```python
from build123d import *

# Parameters (mm, degrees)
BOSS_EXTRUDE1_DEPTH = 0.254
SKETCH2_R           = 4.699
CUT_EXTRUDE1_DEPTH  = 1.254
SKETCH3_W           = 2.54
SKETCH3_H           = 0.635
CUT_EXTRUDE2_DEPTH  = 1.254
CUT_EXTRUDE4_DEPTH  = 1.254
CUT_EXTRUDE5_DEPTH  = 1.254


with BuildPart() as part:
    # Sketch1 → Boss-Extrude1 (new body)
    with BuildSketch(Plane.XY):
        with BuildLine():
            Line((67.21146711, 76.191723231), (8.696654013, 17.676910134))
            Line((8.696654013, 17.676910134), (7.228954972, 14.133571205))
            ThreePointArc((7.228954972, 14.133571205), (14.666587579, 6.075099489), (15.105587123, -4.88230096))
            Line((15.105587123, -4.88230096), (18.648926052, -6.35))
            Line((18.648926052, -6.35), (101.401368334, -6.35))
            ThreePointArc((101.401368334, -6.35), (93.866160503, 38.880636728), (67.21146711, 76.191723231))
        make_face()
        with BuildLine():
            Line((88.672924278, 6.35), (27.86051193, 6.35))
            ThreePointArc((27.86051193, 6.35), (26.399857642, 10.93517908), (24.190484974, 15.210228852))
            Line((24.190484974, 15.210228852), (67.191354125, 58.211098004))
            ThreePointArc((67.191354125, 58.211098004), (82.13289044, 34.020557137), (88.672924278, 6.35))
        make_face(mode=Mode.SUBTRACT)
    extrude(amount=BOSS_EXTRUDE1_DEPTH)

    # Sketch2 → Cut-Extrude1 (cut, through all)
    with BuildSketch(Plane.XY.offset(0.254)):
        with Locations((22.225, 0)):
            Circle(SKETCH2_R)
        with Locations((36.195, 0)):
            Circle(SKETCH2_R)
        with Locations((61.722, 0)):
            Circle(SKETCH2_R)
        with Locations((75.692, 0)):
            Circle(SKETCH2_R)
        with Locations((95.25, 0)):
            Circle(SKETCH2_R)
        with Locations((15.715448212, 15.715448212)):
            Circle(SKETCH2_R)
        with Locations((25.593729945, 25.593729945)):
            Circle(SKETCH2_R)
        with Locations((43.644044748, 43.644044748)):
            Circle(SKETCH2_R)
        with Locations((53.522326482, 53.522326482)):
            Circle(SKETCH2_R)
        with Locations((92.004434954, 24.652514046)):
            Circle(SKETCH2_R)
        with Locations((82.48891971, 47.625)):
            Circle(SKETCH2_R)
        with Locations((67.351920908, 67.351920908)):
            Circle(SKETCH2_R)
    extrude(amount=-CUT_EXTRUDE1_DEPTH, mode=Mode.SUBTRACT)

    # Sketch3 → Cut-Extrude2 (cut, through all)
    with BuildSketch(Plane.XY.offset(0.254)):
        Polygon((15.266435406, 24.246691527), (17.06248663, 26.042742751), (17.511499436, 25.593729945), (15.715448212, 23.797678721), align=None)
        Polygon((44.991083167, 53.971339288), (43.195031942, 52.175288063), (43.644044748, 51.726275257), (45.440095973, 53.522326482), align=None)
        with Locations((29.21, -6.0325)):
            Rectangle(SKETCH3_W, SKETCH3_H)
        with Locations((68.707, -6.0325)):
            Rectangle(SKETCH3_W, SKETCH3_H)
        Polygon((29.230733674, 38.210989795), (31.026784898, 40.007041019), (31.475797704, 39.558028213), (29.67974648, 37.761976989), align=None)
        Polygon((56.845021246, 65.825277367), (55.048970022, 64.029226143), (55.497982828, 63.580213337), (57.294034052, 65.376264561), align=None)
        with Locations((48.9585, -6.0325)):
            Rectangle(SKETCH3_W, SKETCH3_H)
        with Locations((85.471, -6.0325)):
            Rectangle(SKETCH3_W, SKETCH3_H)
        Polygon((99.935462164, 14.437711971), (100.266998693, 11.919442024), (101.526133667, 12.085210288), (101.194597138, 14.603480236), align=None)
        Polygon((93.765504959, 37.464305742), (94.938831965, 37.950313702), (93.966816047, 40.296967714), (92.793489041, 39.810959755), align=None)
        Polygon((79.327792988, 62.471156422), (80.874047017, 60.456038938), (81.88160576, 61.229165953), (80.33535173, 63.244283437), align=None)
        Polygon((13.593916116, 7.005422516), (14.565932035, 4.658768503), (15.739259041, 5.144776462), (14.767243123, 7.491430475), align=None)
    extrude(amount=-CUT_EXTRUDE2_DEPTH, mode=Mode.SUBTRACT)

    # Sketch6 → Cut-Extrude4 (cut, through all)
    with BuildSketch(Plane.XY.offset(0.254)):
        with BuildLine():
            Line((12.392753447, 19.038142977), (22.27103518, 28.91642471))
            ThreePointArc((22.27103518, 28.91642471), (28.91642471, 28.91642471), (28.91642471, 22.27103518))
            Line((28.91642471, 22.27103518), (19.038142977, 12.392753447))
            ThreePointArc((19.038142977, 12.392753447), (12.392753447, 12.392753447), (12.392753447, 19.038142977))
        make_face()
        with BuildLine():
            Line((40.321349984, 46.966739513), (50.199631717, 56.845021246))
            ThreePointArc((50.199631717, 56.845021246), (56.845021246, 56.845021246), (56.845021246, 50.199631717))
            Line((56.845021246, 50.199631717), (46.966739513, 40.321349984))
            ThreePointArc((46.966739513, 40.321349984), (40.321349984, 40.321349984), (40.321349984, 46.966739513))
        make_face()
        with BuildLine():
            Line((22.225, 4.699), (36.195, 4.699))
            ThreePointArc((36.195, 4.699), (40.894, 0), (36.195, -4.699))
            Line((36.195, -4.699), (22.225, -4.699))
            ThreePointArc((22.225, -4.699), (17.526, 0), (22.225, 4.699))
        make_face()
        with BuildLine():
            Line((61.722, 4.699), (75.692, 4.699))
            ThreePointArc((75.692, 4.699), (80.391, 0), (75.692, -4.699))
            Line((75.692, -4.699), (61.722, -4.699))
            ThreePointArc((61.722, -4.699), (57.023, 0), (61.722, 4.699))
        make_face()
        with BuildLine():
            ThreePointArc((99.949, 0), (99.093922449, 13.045962386), (96.543320412, 25.868704739))
            ThreePointArc((96.543320412, 25.868704739), (90.788244261, 29.191399504), (87.465549496, 23.436323353))
            ThreePointArc((87.465549496, 23.436323353), (89.776323642, 11.819277232), (90.551, 0))
            ThreePointArc((90.551, 0), (95.25, -4.699), (99.949, 0))
        make_face()
    extrude(amount=-CUT_EXTRUDE4_DEPTH, mode=Mode.SUBTRACT)

    # Sketch5 → Cut-Extrude5 (cut, through all)
    with BuildSketch(Plane.XY.offset(0.254)):
        with BuildLine():
            Line((70.21145334, 52.434423044), (82.30303448, 61.71261958))
            ThreePointArc((82.30303448, 61.71261958), (89.088033287, 51.435), (94.59621353, 40.420208878))
            Line((94.59621353, 40.420208878), (80.515269058, 34.587690707))
            ThreePointArc((80.515269058, 34.587690707), (75.889806134, 43.815), (70.21145334, 52.434423044))
        make_face()
    extrude(amount=-CUT_EXTRUDE5_DEPTH, mode=Mode.SUBTRACT)


solid = part.part
```
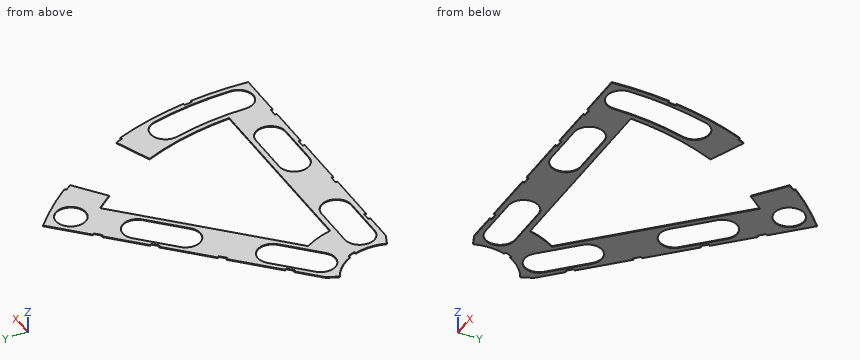
Geometry: final body of the model. Coordinates: model frame, mm. Round coordinates to 2 decimals unless told otherwise and drop trailing zeros. Order: outer loops, then holes, each group sorted by start corner. A loop starts at its lowest first (then second) coordinate and runs counter-clockwise, first axis right, second up. Notation, with made-up numbers: (19.25, 63) -> (72.25, 63) arc R26 ccw to (72.25, 90) -> close; hole circle Ø5 at (5.5, 77). An arc over 180 degrees is marked (long way). Write each question's results on one line, items separated by ' | '.
Q1. Section query A-A (y = 43.5). Output: boundary loops of the cut face in (x, z), and give its area (3 significant figures).
Response values:
outline: (34.52, 0) -> (38.95, 0) -> (38.95, 0.25) -> (34.52, 0.25) -> close; (50.15, 0) -> (52.48, 0) -> (52.48, 0.25) -> (50.15, 0.25) -> close | area: 1.72 mm²
Q2. Section query B-B (z = 0.15). Count the separate pieces of the cut face and the enclosed holes in it, and give its area (3 significant figures).
Response values:
separate pieces: 1 | enclosed holes: 6 | area: 1,540 mm²
Q3. Ray query, line 1 along X through (y, z) = (1, 0.15); line 2 along X through (y, z) = (29.5, 0.05); line 3 along Y through (x, z) = (50, 0.15) (3 decimals). Return the intervals inside material, ascending.
Response values:
line 1: 15.84 to 17.63, 40.79 to 57.13, 80.28 to 90.55, 99.94 to 101.6 | line 2: 20.52 to 22.98, 28.21 to 38.48, 83.86 to 97.22 | line 3: -5.715 to 6.35, 41.02 to 43.355, 56.645 to 58.98
